from build123d import *

# Parameters (mm, degrees)
BOSS_EXTRUDE1_DEPTH = 3.2004
BOSS_EXTRUDE2_START = -3.2004
BOSS_EXTRUDE2_DEPTH = 3.2004
FILLET1_R           = 12.7
CUT_EXTRUDE3_DEPTH  = 3.2004
FILLET2_R           = 2.54
SKETCH9_R           = 2.159
CUT_EXTRUDE4_DEPTH  = 3.2004
CUT_EXTRUDE5_DEPTH  = 3.2004


with BuildPart() as part:
    # Sketch1 → Boss-Extrude1 (new body)
    with BuildSketch(Plane.XY):
        with BuildLine():
            ThreePointArc((-6.790095085, 16.435726481), (57.15, 29.123460788), (121.090095085, 16.435726481))
            ThreePointArc((121.090095085, 16.435726481), (130.735726481, -6.790095085), (107.509904915, -16.435726481))
            ThreePointArc((107.509904915, -16.435726481), (57.15, -6.442730812), (6.790095085, -16.435726481))
            ThreePointArc((6.790095085, -16.435726481), (-16.435726481, -6.790095085), (-6.790095085, 16.435726481))
        make_face()
    extrude(amount=BOSS_EXTRUDE1_DEPTH)

    # Sketch3 → Boss-Extrude2 (add)
    with BuildSketch(Plane.XY.offset(3.2004).offset(BOSS_EXTRUDE2_START)):
        with BuildLine():
            ThreePointArc((96.670173634, 2.329746452), (116.629746452, 17.629826366), (131.929826366, -2.329746452))
            ThreePointArc((131.929826366, -2.329746452), (130.197200475, -12.850112517), (127.798590387, -23.238893209))
            ThreePointArc((127.798590387, -23.238893209), (106.05729345, -35.879818808), (93.416367852, -14.138521872))
            ThreePointArc((93.416367852, -14.138521872), (95.305538892, -5.956206736), (96.670173634, 2.329746452))
        make_face()
    extrude(amount=BOSS_EXTRUDE2_DEPTH)

    # Fillet1
    fillet1_edges = [part.edges().sort_by_distance(p)[0] for p in [
        (94.035611584, -11.705568295, 1.6002),
    ]]
    fillet(fillet1_edges, radius=FILLET1_R)

    # Sketch7 → Cut-Extrude3 (cut)
    with BuildSketch(Plane.XY.offset(3.2004)):
        with BuildLine():
            Line((115.457037918, -18.822354151), (114.672565979, -47.28804272))
            Line((114.672565979, -47.28804272), (104.973448381, -47.020749498))
            Line((104.973448381, -47.020749498), (105.75792032, -18.55506093))
            ThreePointArc((105.75792032, -18.55506093), (110.74112573, -13.839148742), (115.457037918, -18.822354151))
        make_face()
    extrude(amount=-CUT_EXTRUDE3_DEPTH, mode=Mode.SUBTRACT)

    # Fillet2
    fillet2_edges = [part.edges().sort_by_distance(p)[0] for p in [
        (105.286613182, -35.65711589, 1.6002),
        (114.98573078, -35.924409111, 1.6002),
    ]]
    fillet(fillet2_edges, radius=FILLET2_R)

    # Sketch9 → Cut-Extrude4 (cut)
    with BuildSketch(Plane(origin=(0, 0, 0), x_dir=(-1, 0, 0), z_dir=(0, 0, -1))):
        with Locations((-81.171495532, 18.191790938)):
            Circle(SKETCH9_R)
    extrude(amount=-CUT_EXTRUDE4_DEPTH, mode=Mode.SUBTRACT)

    # Sketch10 → Cut-Extrude5 (cut)
    with BuildSketch(Plane(origin=(0, 0, 0), x_dir=(-1, 0, 0), z_dir=(0, 0, -1))):
        with BuildLine():
            Line((-56.134756458, 29.120383205), (25.761959957, 49.584410296))
            Line((25.761959957, 49.584410296), (33.027370327, -48.953888357))
            Line((33.027370327, -48.953888357), (-56.350383293, -6.445154749))
            ThreePointArc((-56.350383293, -6.445154749), (-38.459800898, 11.22980081), (-56.134756458, 29.120383205))
        make_face()
    extrude(amount=-CUT_EXTRUDE5_DEPTH, mode=Mode.SUBTRACT)


solid = part.part
Could you check a few things on this model? Use its own coordinates, in mm. Give positions to 0.01 mm unless a question says otherwise; leave off trailing zeros. Write each loop counter-clockwise with the first axis right and the second up, starting at its lowest first coordinate (ties: lowest second). Pieces come first, ordered by that corner, then holes. Notation, with made-up numbers: (55, 76.25) -> (106, 76.25) arc R18 cw to (106, 99.25) -> close; hole circle Ø10 at (56, -14.75). An arc over 180 degrees is marked (long way). Answer as a JSON object with one key per item and string values.
Q1. Suppose I cut it at A-A on y = 9. Write out the boundary of the cut face in (x, z).
Taken from the geometry:
{"outline": "(38.61, 0) -> (129.64, 0) -> (129.64, 3.2) -> (38.61, 3.2) -> close"}
Q2. Suppose I cut it at B-B on x = 55. Write out the boundary of the cut face in (y, z), then the cut area to 3 significant figures.
Taken from the geometry:
{"outline": "(-6.4, 0) -> (29.08, 0) -> (29.08, 3.2) -> (-6.4, 3.2) -> close", "area": "114 mm²"}
Q3. We'd pull the mould along Y, two halves only. Please class faces 1 (the cylindrical face through (95.633, -28.28, 1.578)), 2 (the cylindrical face through (81.453, 20.332, 1.578)), 3 (the flat face through (86, 5, 0)): released by +Y, released by -Y, zero draft, split by the parting line, or undercut.
Taken from the geometry:
{"face 1": "released by -Y", "face 2": "undercut", "face 3": "zero draft"}
Q4. Will these pins go through, and if not, where does the flat tip stop? pin 1 Ø1.5 at (x, z) = (110, 1) entering from +Y; pin 2 Ø1.5 at (x, y) = (91, -20.5) entering from +Z.
Taken from the geometry:
{"pin 1": "stops at y = 20.81", "pin 2": "passes through"}
Q5. Please list where these lines run through material, in increasing order: L1, parallel to X at y = -25, z = 2; L2, parallel to X at y = -28.5, z = 1.9; L3, parallel to Y at x = 77, z = 2.4.
Taken from the geometry:
{"L1": "x = 93.98 to 105.58, 115.29 to 127.23", "L2": "x = 95.78 to 105.48, 115.19 to 125.44", "L3": "y = -7.95 to 27.94"}
